```python
from build123d import *

# Parameters (mm, degrees)
EXTRUDE_1_DEPTH          = 20
SKETCH_2_R               = 1.5
EXTRUDE_2_DEPTH          = 25
CUT_EXTRUDE_2_DEPTH      = 5
CUT_EXTRUDE_2_DEPTH_BACK = 1
SKETCH_3_R               = 1.5


with BuildPart() as part:
    # 草图1 → 凸台-拉伸1 (new body)
    with BuildSketch(Plane(origin=(0, 0, 0), x_dir=(1, 0, 0), z_dir=(0, 1, 0))):
        Polygon((2.7, 0), (1.35, 2.33826859), (-1.35, 2.33826859), (-2.7, 0), (-1.35, -2.33826859), (1.35, -2.33826859), align=None)
    extrude(amount=EXTRUDE_1_DEPTH)

    # 草图2 → 凸台-拉伸2 (add)
    with BuildSketch(Plane(origin=(0, 0, 0), x_dir=(1, 0, 0), z_dir=(0, 1, 0))):
        with Locations(Location((0, 0, 0), (0, 0, 270))):
            Circle(SKETCH_2_R)
    extrude(amount=EXTRUDE_2_DEPTH)

    # 草图3 → 切除-拉伸2 (cut, two sides: drawn at the far end of the back side and taken through both)
    with BuildSketch(Plane(origin=(0, 0, 0), x_dir=(1, 0, 0), z_dir=(0, 1, 0)).offset(-CUT_EXTRUDE_2_DEPTH_BACK)):
        with Locations(Location((0, 0, 0), (0, 0, 270))):
            Circle(SKETCH_3_R)
    extrude(amount=CUT_EXTRUDE_2_DEPTH + CUT_EXTRUDE_2_DEPTH_BACK, mode=Mode.SUBTRACT)


solid = part.part
```
CAD build for the part. Positions are in the model's coordinates, mm. A direction names the side the tool comes from. Give positions to 0.01 mm unless a question says otherwise; leave off trailing zeros. Loops run counter-clockwise (first coordinate to the right, second up) from the corner with the lowest first, then second, coordinate; pieces in that order, holes last. Notation, with made-up numbers: (-17.75, 51) - (6.25, 51) arc R11 ccw to (6.25, 68) - close; hole circle Ø9 at (-7, -31.75). An arc over 180 degrees is marked (long way). Put each result on its own line as item: value.
Q1. Slice it at A-A (x = 0). Give the cut face in (y, z), plus the area to 3 significant figures.
Filled in:
outline: (0, -2.34) - (20, -2.34) - (20, -1.5) - (25, -1.5) - (25, 1.5) - (20, 1.5) - (20, 2.34) - (0, 2.34) - (0, 1.5) - (5, 1.5) - (5, -1.5) - (0, -1.5) - close
area: 93.5 mm²
Q2. Tool access for faces 4 (the face through (0, 10, -2.338)), 5 (the face through (0.45, 22.46, 1.43)), 6 (the face through (0, 5, 0)): list every direction of +Z, -Z, +X, -X, +Y, -Y with a clear straight run to the whole face (end or side of a thin tool).
Filled in:
face 4: -Z, +X, -X, +Y, -Y
face 5: +Y
face 6: -Y
Q3. Flat gauge pin, fed straight in: pin 1 (1.5 mm diameter, centred on y = 12.5, z = -1.5, fed in from -X). Where does the tip first touch, or does it go through?
Filled in:
pin 1: stops at x = -2.27
Q4. Slice it at D-D (z = 1.15). Give the cut face in (x, y).
Filled in:
outline: (-2.04, 0) - (-0.96, 0) - (-0.96, 5) - (0.96, 5) - (0.96, 0) - (2.04, 0) - (2.04, 20) - (0.96, 20) - (0.96, 25) - (-0.96, 25) - (-0.96, 20) - (-2.04, 20) - close
Q5. Probe line 1 along Z through (x, y) = (0, 3.2); line 2 along Y through (x, z) = (0.75, 1); line 3 along Y through (x, z) = (-1.85, -1.4). List the from-to ranges inside material, lowest first.
Filled in:
line 1: z = -2.34 to -1.5, 1.5 to 2.34
line 2: y = 5 to 25
line 3: y = 0 to 20
Q6. Slice it at B-B (y = 3.5). Give the cut face in (x, z), plus the area to 3 significant figures.
Filled in:
outline: (-2.7, 0) - (-1.35, -2.34) - (1.35, -2.34) - (2.7, 0) - (1.35, 2.34) - (-1.35, 2.34) - close; hole circle Ø3 at (0, 0)
area: 11.9 mm²
Q7. Mould opens along X. For faces 1 (the face through (2.034, 9.86, -1.153)), 2 (the face through (0.45, 2.46, 1.43)), 3 (the face through (-2.034, 9.86, 1.153)) say: pulls with the +X half, pulls with the -X half, needs draft (parallel to the pull), parting line crosses it, or undercut.
Filled in:
face 1: pulls with the +X half
face 2: undercut
face 3: pulls with the -X half
Q8. Slice it at C-C (y = 12.5). Give the cut face in (x, z).
Filled in:
outline: (-2.7, 0) - (-1.35, -2.34) - (1.35, -2.34) - (2.7, 0) - (1.35, 2.34) - (-1.35, 2.34) - close
